Can you work these out from the model? Positions are in its coordinate system, mm. Round coordinates to 2 decimals unless told otherwise and drop trailing zeros. Loops run counter-clockwise (first coordinate to the right, second up) from the corner with the lowest first, then second, coordinate; pieces in that order, holes last.
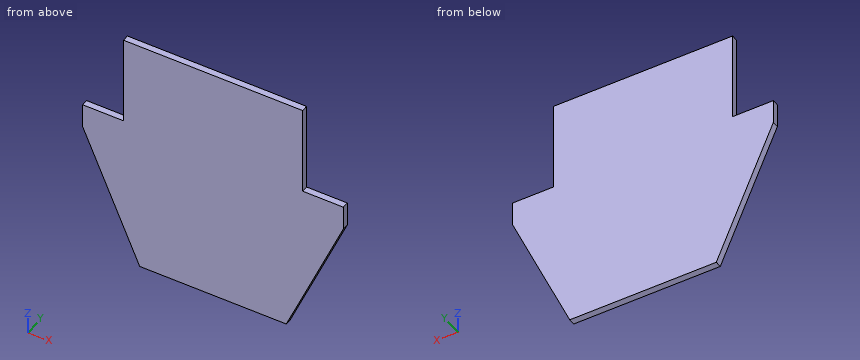
```python
from build123d import *

# Parameters (mm, degrees)
SALIENTE_EXTRUIR1_DEPTH = 2


with BuildPart() as part:
    # Croquis1 → Saliente-Extruir1 (new, symmetric)
    with BuildSketch(Plane(origin=(0, 0, 0), x_dir=(1, 0, 0), z_dir=(0, 1, 0))):
        Polygon((-55, 0), (0, 0), (0, 150), (-45, 150), (-80, 70), (-80, 55), (-55, 55), align=None)
        Polygon((0, 150), (0, 0), (55, 0), (55, 55), (80, 55), (80, 70), (45, 150), align=None)
    extrude(amount=SALIENTE_EXTRUIR1_DEPTH, both=True)


solid = part.part
```
(1) If I drill on line 1 (X direction, y = -1.35, z = -37); line 2 (Z direction, x = -63, y = -1.65); line 3 (Z direction, x = -59, y = 0.15), over which ranges is the centre line in solid material (lowest first)?
(2) For pin 1 (1.2 mm diameter, centred on y = 1, z = -23, fed in from +X); pin 2 (1 mm diameter, centred on y = -1, z = -104.5, fed in from +X) (3 decimals), each with a flat end and sliding along its axis, tell me the tip position at first contact or that it passes through.
(3) Suppose I cut it at B-B (z = -118). Write out the boundary of the cut face in (x, y).
(4) Suppose I cut it at A-A (y = -1.1). Write out the boundary of the cut face in (x, z), then the cut area to 4 significant figures.
(5) Suppose I cut it at C-C (x = -62). Write out the boundary of the cut face in (y, z).
Check result:
1. line 1: x = -55 to 55
1. line 2: z = -108.86 to -55
1. line 3: z = -118 to -55
2. pin 1: stops at x = 55
2. pin 2: stops at x = 65.125
3. outline: (-59, -2) - (59, -2) - (59, 2) - (-59, 2) - close
4. outline: (-80, -70) - (-45, -150) - (45, -150) - (80, -70) - (80, -55) - (55, -55) - (55, 0) - (-55, 0) - (-55, -55) - (-80, -55) - close
4. area: 18,450 mm2
5. outline: (-2, -111.14) - (2, -111.14) - (2, -55) - (-2, -55) - close
